```python
from build123d import *

# Parameters (mm, degrees)
SKETCH_1_W      = 125
SKETCH_1_H      = 10
EXTRUDE_1_DEPTH = 25
M3X0_52_D       = 2.5
M3X0_52_DEPTH   = 12.5
M3X0_52_TIP     = 0.751075774
M3X0_51_D       = 2.5


with BuildPart() as part:
    # Эскиз1 → Бобышка-Вытянуть1 (new body)
    with BuildSketch(Plane.XY):
        with Locations((5.147947656, -18.350453001)):
            Rectangle(SKETCH_1_W, SKETCH_1_H)
    extrude(amount=EXTRUDE_1_DEPTH)

    # Отверстие обработанное метчиком M3x0.52
    with Locations(Plane(origin=(0, 0, 0), x_dir=(-1, 0, 0), z_dir=(0, 0, -1))):
        with Locations((-62.647947656, -18.350453001), (52.352052344, -18.350453001)):
            Hole(M3X0_52_D / 2, depth=M3X0_52_DEPTH)
            with Locations((0, 0, -(M3X0_52_DEPTH + M3X0_52_TIP / 2))):  # 118° drill point
                Cone(0, M3X0_52_D / 2, M3X0_52_TIP, mode=Mode.SUBTRACT)

    # Отверстие обработанное метчиком M3x0.51 (through all)
    with Locations(Plane(origin=(0, -13.350453001, 0), x_dir=(-1, 0, 0), z_dir=(0, 1, 0))):
        with Locations((-44.947947656, 18.5), (-20.947947656, 18.5), (3.052052344, 18.5), (27.052052344, 18.5), (-59.947947656, 18.5)):
            Hole(M3X0_51_D / 2)


solid = part.part
```
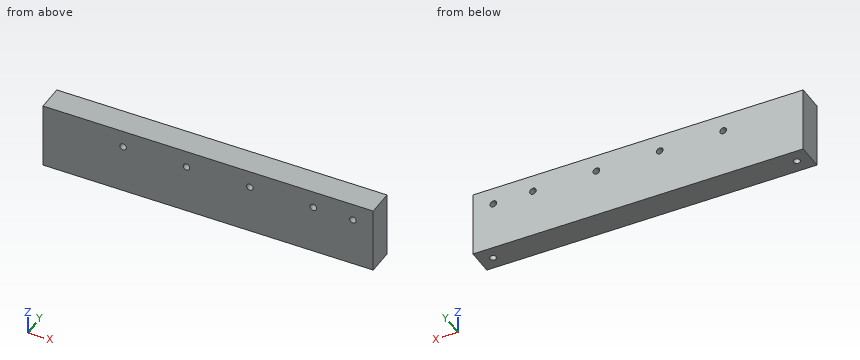
The listing builds one solid part. Answer for the finished solid, in the listing's coordinates (mm). Round coordinates to 2 decimals unless told otherwise and drop trailing zeros. Write each loop counter-clockwise with the first axis right and the second up, starting at its lowest first coordinate (ties: lowest second). Pieces come first, ordered by that corner, then holes. Notation, with made-up numbers: (35.25, 39.25) -> (63.25, 39.25) arc R32 ccw to (63.25, 68.25) -> close; hole circle Ø9 at (-36, -12.5). An arc over 180 degrees is marked (long way). Use CSV: the item, a comma, the result in double quotes. Start each with the question number.
(1) Consider L1, parallel to X at y = -15, z = 18.25; L2, parallel to X at y = -18.5, z = 8; L3, parallel to Z at x = 45, y = -18.5. Determine where each line is inside the solid, lowest interval first. Write a range as from..to.
(2) Each of these flat-tipped pins is pushed along its axis until it touches: pin 1 (1.5 mm diameter, centred on x = -27.05, z = 18.5, fed in from -Y); pin 2 (2 mm diameter, centred on x = 62.65, y = -18.35, fed in from -Z). Where does it stop, or does it pass through?
(3) Section B-B on x = 21 is taken. Give the vertices of the cut face in (y, z).
(4) Section A-A on z = 18.5 is taken. Give the vertices of the cut face in (x, y), then the cut area to 4 significant figures.
A:
1,L1,"x = -57.35..-28.28, -25.83..-4.28, -1.83..19.72, 22.17..43.72, 46.17..58.72, 61.17..67.65"
1,L2,"x = -57.35..-53.59, -51.11..61.41, 63.89..67.65"
1,L3,"z = 0..17.25, 19.75..25"
2,pin 1,"passes through"
2,pin 2,"stops at z = 12.65"
3,outline,"(-23.35, 0) -> (-13.35, 0) -> (-13.35, 17.25) -> (-23.35, 17.25) -> close; (-23.35, 19.75) -> (-13.35, 19.75) -> (-13.35, 25) -> (-23.35, 25) -> close"
4,outline,"(-57.35, -23.35) -> (-28.3, -23.35) -> (-28.3, -13.35) -> (-57.35, -13.35) -> close; (-25.8, -23.35) -> (-4.3, -23.35) -> (-4.3, -13.35) -> (-25.8, -13.35) -> close; (-1.8, -23.35) -> (19.7, -23.35) -> (19.7, -13.35) -> (-1.8, -13.35) -> close; (22.2, -23.35) -> (43.7, -23.35) -> (43.7, -13.35) -> (22.2, -13.35) -> close; (46.2, -23.35) -> (58.7, -23.35) -> (58.7, -13.35) -> (46.2, -13.35) -> close; (61.2, -23.35) -> (67.65, -23.35) -> (67.65, -13.35) -> (61.2, -13.35) -> close"
4,area,"1,125 mm²"
